Here's how the part is built. I have some questions about the finished solid (model axes, mm). Face numbers are marked on the shaded views. A direction names the side the tool comes from. Give positions to 0.01 mm unless a question says otherwise; leave off trailing zeros. Order: outer loops, then holes, each group sorted by start corner. A loop starts at its lowest first (then second) coordinate and runs counter-clockwise, first axis right, second up. Notation, with made-up numbers: M -21,-38 L 10,-38 A18 cw 10,-31 Z; hole C 33.5,23 d3. An arc over 180 degrees is marked long. One line per item, written item: value. Start each with the question number.
from build123d import *

# Parameters (mm, degrees)
F0_W      = 5.842
F0_H      = 12.7
F0_R      = 3.175
F2_DEPTH  = 3.175
F2_TAPER  = -1
F4_DEPTH  = 1.27
F3_R      = 1.524
F5_DEPTH  = 6.35
F6_R      = 1.524
F7_DEPTH  = 6.35
F10_R     = 1.524
F11_DEPTH = 10.414


# Not quite as in the source:
# - a feature of the source that left no trace in its solid (it failed there, or was rolled back) is left out


with BuildPart() as f1:
    # F0 (on Front) → F1 (revolve)
    with BuildSketch(Plane.XZ):
        Polygon((5.842, 12.7), (5.842, 0), (66.294, 0), (66.294, 12.7), (56.134, 12.7), (56.134, 10.16), (10.16, 10.16), (10.16, 12.7), align=None)
        with Locations((2.921, 6.35)):
            Rectangle(F0_W, F0_H)
    revolve(axis=Axis((33.147, 0, 0), (-1, 0, 0)))

    # F0 (on Front) → F2 (join, symmetric)
    with BuildSketch(Plane.XZ):
        with BuildLine():
            Line((5.842, 0), (0, 0))
            Line((0, 0), (-0.9398, 0))
            ThreePointArc((-0.9398, 0), (-3.1957909266, -4.5493385486), (-8.1826630726, -5.5069827884))
            Line((-8.1826630726, -5.5069827884), (5.842, -9.398))
            Line((5.842, -9.398), (5.842, 0))
        make_face()
        with BuildLine():
            ThreePointArc((-8.1826630726, -5.5069827884), (-3.1957909266, -4.5493385486), (-0.9398, 0))
            ThreePointArc((-0.9398, 0), (-4.5919612295, 5.3297205562), (-10.8806298187, 3.8475430269))
            ThreePointArc((-10.8806298187, 3.8475430269), (-12.1459778134, -1.5837270034), (-8.1826630726, -5.5069827884))
        make_face()
        with Locations((-6.6548, 0)):
            Circle(F0_R, mode=Mode.SUBTRACT)
        with BuildLine():
            Line((-0.9398, 0), (0, 0))
            Line((0, 0), (0, 12.7))
            Line((0, 12.7), (5.842, 12.7))
            Line((5.842, 12.7), (5.842, 15.24))
            Line((5.842, 15.24), (-0.508, 15.24))
            Line((-0.508, 15.24), (-10.8806298187, 3.8475430269))
            ThreePointArc((-10.8806298187, 3.8475430269), (-4.5919612295, 5.3297205562), (-0.9398, 0))
        make_face()
    extrude(amount=F2_DEPTH, both=True, taper=F2_TAPER)

    # F3 (on face) → F4 (join)
    with BuildSketch(Plane.YZ.offset(66.294)):
        with BuildLine():
            ThreePointArc((-5.08, 11.6397422652), (0, 12.7), (5.08, 11.6397422652))
            Line((5.08, 11.6397422652), (5.08, 15.24))
            Line((5.08, 15.24), (-5.08, 15.24))
            Line((-5.08, 15.24), (-5.08, 11.6397422652))
        make_face()
    extrude(amount=-F4_DEPTH)

    # F3 (on face) → F5 (join)
    with BuildSketch(Plane.YZ.offset(66.294)):
        with BuildLine():
            ThreePointArc((-5.08, 11.6397422652), (0, 12.7), (5.08, 11.6397422652))
            Line((5.08, 11.6397422652), (5.08, 15.24))
            Line((5.08, 15.24), (-5.08, 15.24))
            Line((-5.08, 15.24), (-5.08, 11.6397422652))
        make_face()
        with BuildLine():
            ThreePointArc((-5.08, 0), (0, 5.08), (5.08, 0))
            Line((5.08, 0), (5.08, 11.6397422652))
            ThreePointArc((5.08, 11.6397422652), (0, 12.7), (-5.08, 11.6397422652))
            Line((-5.08, 11.6397422652), (-5.08, 0))
        make_face()
        with BuildLine():
            ThreePointArc((-5.08, 0), (0, -5.08), (5.08, 0))
            ThreePointArc((5.08, 0), (0, 5.08), (-5.08, 0))
        make_face()
        Circle(F3_R, mode=Mode.SUBTRACT)
        Circle(F3_R)
    extrude(amount=F5_DEPTH)

    # F6 (on face) → F7 (cut, through all)
    with BuildSketch(Plane.YZ.offset(72.644)):
        Circle(F6_R)
    extrude(amount=-F7_DEPTH, mode=Mode.SUBTRACT)

    # F10 (on face) → F11 (cut)
    with BuildSketch(Plane.XY.offset(15.24)):
        with Locations((68.834, 0)):
            Circle(F10_R)
    extrude(amount=-F11_DEPTH, mode=Mode.SUBTRACT)


solid = f1.part
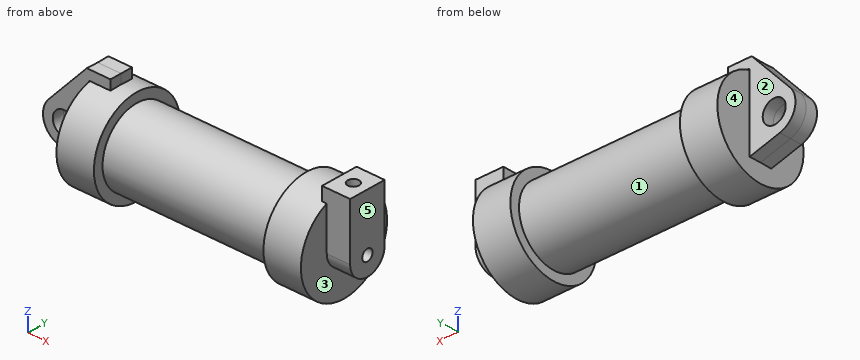
Item 1: I want a section at A-A on x = 62. Write out the boundary of the cut face in (y, z), plus the area to 3 significant figures.
Item 2: Please list where these lines run through material, in increasing order: probe 1 along X at (y, z) = (-9, -5.25); probe 2 along Z at (x, y) = (68.25, 0); probe 3 along X at (y, z) = (5.75, 0.75). Write a range as [from, to].
Item 3: We'd pull the mould along X, two halves only. Please class the marked faces 1, 2 and 3: +X half, -X half, draft (parallel to the pull), parting line (faces both ways), or undercut.
Item 4: I want a section at C-C on z = -9. Write out the boundary of the cut face in (x, y), plus the area to 3 significant figures.
Item 5: Will these pins go through, and if not, where does the flat tip stop? P1, Ø2.5, axis at y = 0, z = 0, coming from the +X side; P2, Ø12, axis at y = -10, z = -1.5, coming from the -X side; P3, Ø5.5, axis at x = 0, z = 7.5, coming from the +Y side.
Item 6: I want a section at D-D on x = 26. Write out the boundary of the cut face in (y, z).
Item 7: I want a section at B-B on y = -8.75. Write out the boundary of the cut face in (x, z), plus the area to 3 significant figures.
Item 8: For the marked faces 4 and 5, which set-ups out of +Z, -Z, +X, -X, +Y, -Y let a thin tool reach every point of the face, with its end or its side?
Answer below:
1. outline: C 0,0 d25.4
1. area: 507 mm²
2. probe 1: x = [0, 10.16], [56.13, 66.29]
2. probe 2: z = [-5.08, -1.52], [1.52, 4.83]
2. probe 3: x = [0, 66.29]
3. face 1: undercut
3. face 2: draft
3. face 3: +X half
4. outline: M 0,-8.96 L 10.16,-8.96 L 10.16,-4.71 L 56.13,-4.71 L 56.13,-8.96 L 66.29,-8.96 L 66.29,8.96 L 56.13,8.96 L 56.13,4.71 L 10.16,4.71 L 10.16,8.96 L 0,8.96 Z
4. area: 798 mm²
5. P1: stops at x = 66.29
5. P2: stops at x = 0
5. P3: stops at y = 11.78
6. outline: C 0,0 d20.32
7. outline: M 0,-9.2 L 10.16,-9.2 L 10.16,-5.16 L 56.13,-5.16 L 56.13,-9.2 L 66.29,-9.2 L 66.29,9.2 L 56.13,9.2 L 56.13,5.16 L 10.16,5.16 L 10.16,9.2 L 0,9.2 Z
7. area: 849 mm²
8. face 4: -Z, -X
8. face 5: +Z, -Z, +X, +Y, -Y
